The model under review builds one solid part; all positions refer to its coordinate system, in mm. A direction names the side the tool comes from. Round coordinates to 2 decimals unless told otherwise and drop trailing zeros. Order: outer loops, then holes, each group sorted by start corner. A loop starts at its lowest first (then second) coordinate and runs counter-clockwise, first axis right, second up. Notation, with made-up numbers: (86.25, 57.5) -> (102.25, 57.5) arc R15 ccw to (102.25, 86.5) -> close; hole circle Ø6 at (42, 29.5). An arc over 180 degrees is marked (long way). Return JSON: item names as keys, results as strings. Group by question number.
from build123d import *

# Parameters (mm, degrees)
F1_DEPTH        = 22
F0_W            = 42
F0_H            = 110
F2_DEPTH        = 2
F3_W            = 20
F3_H            = 7
F4_DEPTH        = 25
F6_W            = 20
F6_H            = 7
F7_DEPTH        = 25
F9_D            = 10
F9_CSINK_D      = 15
F9_CSINK_ANGLE  = 90
F11_D           = 10
F11_CSINK_D     = 15
F11_CSINK_ANGLE = 90
F13_D           = 10
F13_CSINK_D     = 15
F13_CSINK_ANGLE = 90
F15_D           = 10
F15_CSINK_D     = 15
F15_CSINK_ANGLE = 90


with BuildPart() as f1:
    # F0 (on Top) → F1 (new body)
    with BuildSketch(Plane.XY):
        Polygon((-12.002976, 0), (0, 0), (0, 110), (42, 110), (42, 0), (55.389886, 0), (55.389886, 120.241073), (-12.002976, 120.241073), align=None)
    extrude(amount=F1_DEPTH)

    # F0 (on Top) → F2 (join)
    with BuildSketch(Plane.XY):
        with Locations((21, 55)):
            Rectangle(F0_W, F0_H)
        Polygon((-12.002976, 0), (0, 0), (0, 110), (42, 110), (42, 0), (55.389886, 0), (55.389886, 120.241073), (-12.002976, 120.241073), align=None)
    extrude(amount=-F2_DEPTH)

    # F3 (on face) → F4 (join)
    with BuildSketch(Plane.YZ.offset(55.389886)):
        with Locations((15, 18.5)):
            Rectangle(F3_W, F3_H)
        with Locations((105, 18.5)):
            Rectangle(F3_W, F3_H)
    extrude(amount=F4_DEPTH)

    # F6 (on face) → F7 (join)
    with BuildSketch(Plane(origin=(-12.002976, 0, 0), x_dir=(0, -1, 0), z_dir=(-1, 0, 0))):
        with Locations((-105.241073, 18.5)):
            Rectangle(F6_W, F6_H)
        with Locations((-15.041073, 18.5)):
            Rectangle(F6_W, F6_H)
    extrude(amount=F7_DEPTH)

    # F9 (through all)
    with Locations(Plane(origin=(0, 0, 15), x_dir=(1, 0, 0), z_dir=(0, 0, -1))):
        with Locations((67.889886, -105)):
            CounterSinkHole(F9_D / 2, F9_CSINK_D / 2, counter_sink_angle=F9_CSINK_ANGLE)

    # F11 (through all)
    with Locations(Plane(origin=(0, 0, 15), x_dir=(1, 0, 0), z_dir=(0, 0, -1))):
        with Locations((67.889886, -15)):
            CounterSinkHole(F11_D / 2, F11_CSINK_D / 2, counter_sink_angle=F11_CSINK_ANGLE)

    # F13 (through all)
    with Locations(Plane(origin=(0, 0, 15), x_dir=(1, 0, 0), z_dir=(0, 0, -1))):
        with Locations((-24.502976, -15.041073)):
            CounterSinkHole(F13_D / 2, F13_CSINK_D / 2, counter_sink_angle=F13_CSINK_ANGLE)

    # F15 (through all)
    with Locations(Plane(origin=(0, 0, 15), x_dir=(1, 0, 0), z_dir=(0, 0, -1))):
        with Locations((-24.502976, -105.241073)):
            CounterSinkHole(F15_D / 2, F15_CSINK_D / 2, counter_sink_angle=F15_CSINK_ANGLE)


solid = f1.part
Item 1: Consider section B-B on z = 6.25. State the section outline as (x, y) points.
Item 2: For faces 5 (the face through (55.39, 59, 8)), 6 (the face through (-16, 105, 15)), 7 (the face through (0, 54, 11)), list the 3-axis set-ups (+Z, -Z, +X, -X, +Y, -Y) from which the entire face can be reached by the end or side of a thin tool; tool diameter is ignored.
Item 3: Consider section A-A on y = 47. State the section outline as (x, z) points.
Item 4: Wall thickness on line 1 along X through (y, z) = (105, 20.8); line 2 along X through (y, z) = (55.5, 9); line 3 along Y through (x, z) = (68, 16.5): over which ranges is each line inside the solid? List them lowest first.
Item 5: Consider section C-C on x = -22. Give the number of separate pieces and of enclosed holes in the cut face, plus the area to 3 significant figures.
Item 6: The part is to be moulded in two halves that separate along X. For faces 1 (the face through (80.39, 15, 19)), 2 (the face through (68, 95, 18)), 3 (the face through (-20.82, 11.66, 19.78)), 4 (the face through (-37.003, 15, 19)), say which applies: +X half, -X half, draft (parallel to the pull), parting line (faces both ways), or undercut.
Item 7: Insertion check: pin 1 Ø6 at (y, z) = (70.5, 12.5) entering from -X; pin 2 Ø9 at (x, y) = (67.89, 105) entering from -Z; pin 3 Ø5.5 at (x, z) = (68.5, 17) entering from -Y; pin 4 Ø3.5 at (x, z) = (-19, 18.5) entering from +Y. Each pin has a flat end and moves straight along its axis. Give the tip position at first contact, or say it passes through.
Values:
{
 "1": {"outline": "(-12, 0) -> (0, 0) -> (0, 110) -> (42, 110) -> (42, 0) -> (55.39, 0) -> (55.39, 120.24) -> (-12, 120.24) -> close"},
 "2": {"face 5": "-Z, +X", "face 6": "-Z, -X, +Y, -Y", "face 7": "+Z, -Y"},
 "3": {"outline": "(-12, -2) -> (55.39, -2) -> (55.39, 22) -> (42, 22) -> (42, 0) -> (0, 0) -> (0, 22) -> (-12, 22) -> close"},
 "4": {"line 1": "-37 to -29.5, -19.51 to 0, 42 to 62.89, 72.89 to 80.39", "line 2": "-12 to 0, 42 to 55.39", "line 3": "5 to 9, 21 to 25, 95 to 99, 111 to 115"},
 "5": {"separate pieces": "4", "enclosed holes": "0", "area": "145 mm^2"},
 "6": {"face 1": "+X half", "face 2": "draft", "face 3": "undercut", "face 4": "-X half"},
 "7": {"pin 1": "x = -12", "pin 2": "through", "pin 3": "y = 5", "pin 4": "y = 115.24"}
}
